Can you work these out from the model? Positions are in its coordinate system, mm. Round coordinates to 2 decimals unless told otherwise and drop trailing zeros. Write each loop counter-clockwise with the first axis right and the second up, starting at its lowest first coordinate (ties: lowest second). Pieces come first, ordered by that corner, then holes. Notation, with made-up numbers: (22, 69) -> (59, 69) arc R19 ccw to (59, 106) -> close; hole circle Ø5 at (56, 49). An arc over 180 degrees is marked (long way). Use CSV: the item, a comma, the result in double quotes.
```python
from build123d import *

# Parameters (mm, degrees)
SKETCH1_W           = 28
SKETCH1_H           = 6
BOSS_EXTRUDE1_DEPTH = 12.5
SKETCH2_R           = 1
CUT_EXTRUDE1_DEPTH  = 435
SKETCH3_R           = 2.25
CUT_EXTRUDE2_DEPTH  = 20.704060495


with BuildPart() as part:
    # Sketch1 → Boss-Extrude1 (new, symmetric)
    with BuildSketch(Plane.XY):
        with Locations((0, 3)):
            Rectangle(SKETCH1_W, SKETCH1_H)
    extrude(amount=BOSS_EXTRUDE1_DEPTH, both=True)

    # Sketch2 → Cut-Extrude1 (cut)
    with BuildSketch(Plane.XY.offset(12.5)):
        with Locations((-4, 0)):
            Circle(SKETCH2_R)
        with Locations((4, 0)):
            Circle(SKETCH2_R)
    extrude(amount=-CUT_EXTRUDE1_DEPTH, mode=Mode.SUBTRACT)

    # Sketch3 → Cut-Extrude2 (cut, through all)
    with BuildSketch(Plane(origin=(0, 6, 0), x_dir=(1, 0, 0), z_dir=(0, 1, 0))):
        with Locations(Location((-10, 7.5, 0), (0, 0, 270))):
            Circle(SKETCH3_R)
        with Locations(Location((-10, -7.5, 0), (0, 0, 270))):
            Circle(SKETCH3_R)
        with Locations(Location((10, -7.5, 0), (0, 0, 270))):
            Circle(SKETCH3_R)
        with Locations(Location((10, 7.5, 0), (0, 0, 270))):
            Circle(SKETCH3_R)
    extrude(amount=-CUT_EXTRUDE2_DEPTH, mode=Mode.SUBTRACT)


solid = part.part
```
Q1. Suppose I cut it at A-A (x = -10). Write out the boundary of the cut face in (y, z).
Resolved:
outline,"(0, -12.5) -> (6, -12.5) -> (6, -9.75) -> (0, -9.75) -> close; (0, -5.25) -> (6, -5.25) -> (6, 5.25) -> (0, 5.25) -> close; (0, 9.75) -> (6, 9.75) -> (6, 12.5) -> (0, 12.5) -> close"
Q2. If we mould it in two halves opening along X, with no side actions, what happens to faces 1 (the face through (-4, 1, 0)), 2 (the face through (-14, 3, 0)), 3 (the face through (0, 0, 0))? For each: released by +X, released by -X, zero draft, split by the parting line, or undercut.
Resolved:
face 1,"undercut"
face 2,"released by -X"
face 3,"zero draft"
Q3. Please list where these lines run through material, in increasing order: probe 1 along X at (y, z) = (4.2, 7.5); probe 2 along X at (y, z) = (4.35, -8.25); probe 3 along Z at (x, y) = (11.5, 1.2).
Resolved:
probe 1,"x = -14 to -12.25, -7.75 to 7.75, 12.25 to 14"
probe 2,"x = -14 to -12.12, -7.88 to 7.88, 12.12 to 14"
probe 3,"z = -12.5 to -9.18, -5.82 to 5.82, 9.18 to 12.5"
Q4. Suppose I cut it at D-D (z = -10.5). Write out the boundary of the cut face in (x, y).
Resolved:
outline,"(-14, 0) -> (-5, 0) arc R1 cw to (-3, 0) -> (3, 0) arc R1 cw to (5, 0) -> (14, 0) -> (14, 6) -> (-14, 6) -> close"
Q5. Will this pin go through, and if not, where does the flat tip stop? P1, Ø2.5, axis at x = -10, z = 7.5, coming from the +Y side.
Resolved:
P1,"passes through"
Q6. Suppose I cut it at B-B (z = -7.5). Write out the boundary of the cut face in (x, y).
Resolved:
outline,"(-14, 0) -> (-12.25, 0) -> (-12.25, 6) -> (-14, 6) -> close; (-7.75, 0) -> (-5, 0) arc R1 cw to (-3, 0) -> (3, 0) arc R1 cw to (5, 0) -> (7.75, 0) -> (7.75, 6) -> (-7.75, 6) -> close; (12.25, 0) -> (14, 0) -> (14, 6) -> (12.25, 6) -> close"
Q7. Suppose I cut it at C-C (y = 4.45). Write out the boundary of the cut face in (x, z).
Resolved:
outline,"(-14, -12.5) -> (14, -12.5) -> (14, 12.5) -> (-14, 12.5) -> close; hole circle Ø4.5 at (-10, -7.5); hole circle Ø4.5 at (-10, 7.5); hole circle Ø4.5 at (10, -7.5); hole circle Ø4.5 at (10, 7.5)"
